from build123d import *

# Parameters (mm, degrees)
SKETCH_1_R          = 2
EXTRUDE_1_DEPTH     = 98
SKETCH_4_W          = 0.6
SKETCH_4_H          = 4.591769547
CUT_EXTRUDE_1_DEPTH = 6
SKETCH_5_W          = 0.6
SKETCH_5_H          = 4.626337449
CUT_EXTRUDE_2_DEPTH = 6
FILLET_1_R          = 0.1


with BuildPart() as part:
    # 草图1 → 凸台-拉伸1 (new body)
    with BuildSketch(Plane.XY):
        Circle(SKETCH_1_R)
    extrude(amount=-EXTRUDE_1_DEPTH)

    # 草图2 → 旋转1 (revolve)
    with BuildSketch(Plane(origin=(0, 0, 0), x_dir=(1, 0, 0), z_dir=(0, 1, 0))):
        Polygon((2, 98), (2, 95), (2.2, 95), (2.2, 96), align=None)
    revolve(axis=Axis((0, 0, -98.400889699), (0, 0, 1)))

    # 草图3 → 旋转2 (revolve)
    with BuildSketch(Plane(origin=(0, 0, 0), x_dir=(1, 0, 0), z_dir=(0, 1, 0)), mode=Mode.PRIVATE) as revolve_2_sk:
        Polygon((2, 0), (2, 3), (2.2, 3), (2.2, 2), align=None)
    revolve(revolve_2_sk.sketch.rotate(Axis((0, 0, 0.764121939), (0, 0, -1)), 180), axis=Axis((0, 0, 0.764121939), (0, 0, -1)))

    # 草图4 → 切除-拉伸1 (cut)
    with BuildSketch(Plane.XY):
        with Locations((0, -0.031687242)):
            Rectangle(SKETCH_4_W, SKETCH_4_H)
    extrude(amount=-CUT_EXTRUDE_1_DEPTH, mode=Mode.SUBTRACT)

    # 草图5 → 切除-拉伸2 (cut)
    with BuildSketch(Plane(origin=(0, 0, -98), x_dir=(-1, 0, 0), z_dir=(0, 0, -1))):
        with Locations((0, -0.054732511)):
            Rectangle(SKETCH_5_W, SKETCH_5_H)
    extrude(amount=-CUT_EXTRUDE_2_DEPTH, mode=Mode.SUBTRACT)

    # 圆角1
    fillet_1_edges = [part.edges().sort_by_distance(p)[0] for p in [
        (0.3, 0, -98),
        (2, 0, -98),
        (-0.3, 0, -98),
        (-2, 0, -98),
        (-2, 0, 0),
        (-0.3, 0, 0),
        (2, 0, 0),
        (0.3, 0, 0),
    ]]
    fillet(fillet_1_edges, radius=FILLET_1_R)


solid = part.part
Source: CAD feature listing. Evaluate the final solid. Frame: model axes, mm. A direction names the side the tool comes from. Coordinates: 2 decimals unless noted, no trailing zeros. Loops run counter-clockwise (first coordinate to the right, second up) from the corner with the lowest first, then second, coordinate; pieces in that order, holes last. Notation, with made-up numbers: (51.5, 8) -> (109.5, 8) arc R30 cw to (109.5, 35) -> close; hole circle Ø8 at (44, 0). An arc over 180 degrees is marked (long way). Answer in a Markdown table with one row per item. Add a question column.
Q1. Section B-B on z = -77.5. Return the cut outline in (x, y), and give its area (3 significant figures).
Q2. Contact query for flat-ended pins moving along their axis: pin 1 Ø2 at (x, y) = (-1, -1) entering from +Z; pin 2 Ø2 at (x, z) = (1, -24) entering from -Y; pin 3 Ø1.3 at (y, z) = (-1, -95) entering from +X. Output: stop coordinate, or through.
Q3. Ray query, line 1 along Z through (x, y) = (0.8, 1.75); line 2 along Z through (x, y) = (-0.15, 1.4); line 3 along Y through (x, z) = (0.7, -56.5). Return the intervals inside material, ascending.
Q4. Reachability of faces 1 (the face through (-2.1, 0, -97)), 2 (the face through (-0.3, 0, -3)), 3 (the face through (0.3, 0, -95)) from +Z, -Z, +X, -X, +Y, -Y: full face, straight path, thin tool, end or side. Return the list, or none.
Computed values:
| question | item | result |
|---|---|---|
| 1 | outline | circle Ø4 at (0, 0) |
| 1 | area | 12.6 mm^2 |
| 2 | pin 1 | stops at z = 0 |
| 2 | pin 2 | stops at y = -2 |
| 2 | pin 3 | stops at x = 2.17 |
| 3 | line 1 | z = -98 to 0 |
| 3 | line 2 | z = -92 to -6 |
| 3 | line 3 | y = -1.87 to 1.87 |
| 4 | face 1 | -Z, -X |
| 4 | face 2 | +Z, +Y, -Y |
| 4 | face 3 | -Z, +Y, -Y |
